The drawing under review shows one solid part. Ordinate dimensions are in mm from its lowest x, y, z. A direction names the side the tool comes from. Coordinates: 2 decimals unless noted, no trailing zeros. Write each loop counter-clockwise with the first axis right and the second up, starting at its lowest first coordinate (ties: lowest second). Pieces come first, ordered by that corner, then holes. Notation, with made-up numbers: M 65.5,10 L 103.5,10 A29 ccw 103.5,49 Z; hole C 32,15.25 d8. An arc over 180 degrees is marked long. Write each question's results on one line, items separated by ' | '. Start each with the question number.
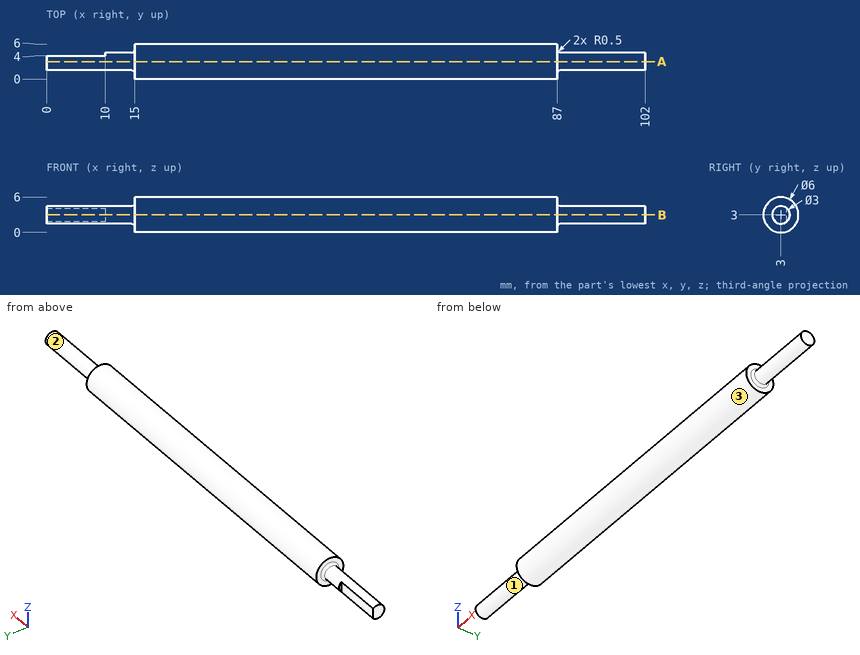
Item 1: We need section B-B on z = 3. State the section outline as (x, y) points, then the cut area to 3 significant figures.
Item 2: Wall thickness on L1, parallel to Z at x = 19.5, y = 2.8; L2, parallel to X at y = 5, z = 1; L3, parallel to Y at x = 88, z = 3.25: over which ranges is each line inside the solid? List them lowest first.
Item 3: Insertion check: pin 1 Ø0.7 at (x, z) = (3.5, 2.5) entering from +Y; pin 2 Ø1.8 at (y, z) = (3, 3.5) entering from -X; pin 3 Ø1 at (x, y) = (51, 1) entering from +Z. Each pin has a flat end and moves straight along its axis. Give the tip position at first contact, or say it passes through.
Item 4: For the marked faces 1, 2 and 3, list the 3-axis set-ups (+Z, -Z, +X, -X, +Y, -Y) from which the entire face can be reached by the end or side of a thin tool; tool diameter is ignored.
Item 5: We need section A-A on y = 3. State the section outline as (x, z) points.
Answer:
1) outline: M 0,1.5 L 14.5,1.5 A0.5 cw 15,1 L 15,0 L 87,0 L 87,1 A0.5 cw 87.5,1.5 L 102,1.5 L 102,4.5 L 87.5,4.5 A0.5 cw 87,5 L 87,6 L 15,6 L 15,5 A0.5 cw 14.5,4.5 L 10,4.5 L 10,4 L 0,4 Z | area: 517 mm^2
2) L1: z = 0.01 to 5.99 | L2: x = 15 to 87 | L3: y = 1.52 to 4.48
3) pin 1: stops at y = 4 | pin 2: stops at x = 0 | pin 3: stops at z = 5.6
4) face 1: -X | face 2: +X | face 3: +X, -X
5) outline: M 0,1.5 L 14.5,1.5 A0.5 cw 15,1 L 15,0 L 87,0 L 87,1 A0.5 cw 87.5,1.5 L 102,1.5 L 102,4.5 L 87.5,4.5 A0.5 cw 87,5 L 87,6 L 15,6 L 15,5 A0.5 cw 14.5,4.5 L 0,4.5 Z
